Here's how the part is built. I have some questions about the finished solid (model axes, mm). Coordinates: 2 decimals unless noted, no trailing zeros. Loops run counter-clockwise (first coordinate to the right, second up) from the corner with the lowest first, then second, coordinate; pieces in that order, holes last. Notation, with made-up numbers: (70, 61) - (113, 61) arc R8 cw to (113, 70) - close; hole circle Ø3 at (-26.5, 35). An arc over 180 degrees is marked (long way). Use a Markdown table: item, result.
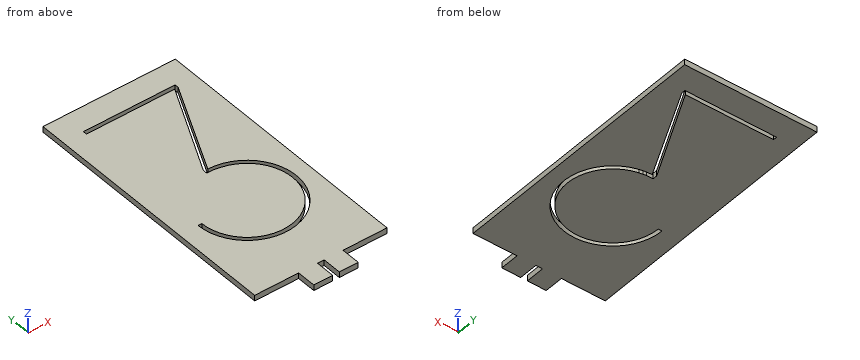
```python
from build123d import *

# Parameters (mm, degrees)
SKIZZE1_W                       = 35
SKIZZE1_H                       = 75
AUFSATZ_LINEAR_AUSTRAGEN1_DEPTH = 1.5
SKIZZE2_W                       = 11.63
SKIZZE2_H                       = 5
SKIZZE2_W_2                     = 11.62
SKIZZE2_W_3                     = 1.75
SCHNITT_LINEAR_AUSTRAGEN1_DEPTH = 1.5
SCHNITT_LINEAR_AUSTRAGEN4_DEPTH = 20


with BuildPart() as part:
    # Skizze1 → Aufsatz-Linear austragen1 (new body)
    with BuildSketch(Plane.XY):
        with Locations((17.5, 37.5)):
            Rectangle(SKIZZE1_W, SKIZZE1_H)
    extrude(amount=AUFSATZ_LINEAR_AUSTRAGEN1_DEPTH)

    # Skizze2 → Schnitt-Linear austragen1 (cut)
    with BuildSketch(Plane.XY.offset(1.5)):
        with Locations((5.815, 2.5)):
            Rectangle(SKIZZE2_W, SKIZZE2_H)
        with Locations((29.19, 2.5)):
            Rectangle(SKIZZE2_W_2, SKIZZE2_H)
        with Locations((17.505, 2.5)):
            Rectangle(SKIZZE2_W_3, SKIZZE2_H)
    extrude(amount=-SCHNITT_LINEAR_AUSTRAGEN1_DEPTH, mode=Mode.SUBTRACT)

    # Skizze9 → Schnitt-Linear austragen4 (cut)
    with BuildSketch(Plane.XY.offset(1.5)):
        with BuildLine():
            Line((18, 43), (29.734930419, 67.5))
            Line((29.734930419, 67.5), (29.734930419, 68.5))
            Line((29.734930419, 68.5), (5.5, 68.5))
            Line((5.5, 68.5), (5.5, 67.5))
            Line((5.5, 67.5), (28.826499189, 67.5))
            Line((28.826499189, 67.5), (17, 43.230685214))
            Line((17, 43.230685214), (17, 42.069041261))
            Line((17, 42.069041261), (18.731597041, 42.069041261))
            Line((18.731597041, 42.069041261), (19.547222411, 41.915420677))
            Line((19.547222411, 41.915420677), (20.52804755, 41.730685214))
            ThreePointArc((20.52804755, 41.730685214), (25.538681231, 20.663604266), (6, 30))
            Line((6, 30), (5, 30))
            ThreePointArc((5, 30), (27.192388155, 20.807611845), (18, 43))
        make_face()
    extrude(amount=-SCHNITT_LINEAR_AUSTRAGEN4_DEPTH, mode=Mode.SUBTRACT)


solid = part.part
```
Q1. I want a section at B-B, the plane y = 37. Write out the boundary of the cut face in (x, z), then the cut area to 3 significant figures.
Check values:
| item | result |
|---|---|
| outline | (0, 0) - (27.75, 0) - (27.75, 1.5) - (0, 1.5) - close; (28.95, 0) - (35, 0) - (35, 1.5) - (28.95, 1.5) - close |
| area | 50.7 mm^2 |
Q2. I want a section at C-C, the plane y = 45. Write out the boundary of the cut face in (x, z), then the cut area to 3 significant figures.
Check values:
| item | result |
|---|---|
| outline | (0, 0) - (17.86, 0) - (17.86, 1.5) - (0, 1.5) - close; (18.96, 0) - (35, 0) - (35, 1.5) - (18.96, 1.5) - close |
| area | 50.9 mm^2 |
Q3. Please list where these lines run through material, in increasing order: L1, parallel to X at y = 29.5, z = 0.7; L2, parallel to Y at x = 16.5, z = 0.2; L3, parallel to Y at x = 7.5, z = 0.65. Write a range as from..to.
Check values:
| item | result |
|---|---|
| L1 | 0..5.01, 6.01..29.99, 30.99..35 |
| L2 | 0..17.09, 18.09..67.5, 68.5..75 |
| L3 | 5..22.34, 24.19..67.5, 68.5..75 |
Q4. I want a section at A-A, the plane z = 0.9. Write out the boundary of the cut face in (x, y), then the cut area to 3 significant figures.
Check values:
| item | result |
|---|---|
| outline | (0, 5) - (11.63, 5) - (11.63, 0) - (16.63, 0) - (16.63, 5) - (18.38, 5) - (18.38, 0) - (23.38, 0) - (23.38, 5) - (35, 5) - (35, 75) - (0, 75) - close; hole (5, 30) arc R13 ccw (long way) to (18, 43) - (29.73, 67.5) - (29.73, 68.5) - (5.5, 68.5) - (5.5, 67.5) - (28.83, 67.5) - (17, 43.23) - (17, 42.07) - (18.73, 42.07) - (20.53, 41.73) arc R12 cw (long way) to (6, 30) - close |
| area | 2,390 mm^2 |
Q5. Will these pins go through, and if not, where does the flat tip stop? P1, Ø0.8, axis at y = 68, z = 1, coming from the -X side; P2, Ø0.8, axis at y = 2.5, z = 0.5, coming from the -X side; P3, Ø0.8, axis at y = 2, z = 0.5, coming from the +X side; P4, Ø0.8, axis at x = 7, z = 1, coming from the -Y side.
Check values:
| item | result |
|---|---|
| P1 | x = 0 |
| P2 | x = 11.63 |
| P3 | x = 23.38 |
| P4 | y = 5 |
